Geometry: final body of the model. Coordinates: model frame, mm. A direction names the side the tool comes from. Coordinates: 2 decimals unless noted, no trailing zeros. Write each loop counter-clockwise with the first axis right and the second up, starting at its lowest first coordinate (ties: lowest second). Pieces come first, ordered by that corner, then holes. Notation, with made-up numbers: (-34, 11) - (-28, 11) arc R12 ccw to (-28, 22) - close; hole circle Ø10 at (38, -5.75). An arc over 180 degrees is marked (long way). Answer as a JSON object with one key per item and string values. Group by question number.
Item 1: Line query: line 1 along X through (y, z) = (175, 3.9); line 2 along Y through (x, z) = (166, 1.9); line 3 along Y through (x, z) = (156, 4.15). Output: solid intervals per line, ascending. Write a range as from..to.
Item 2: Mould query, pull axis X, two halves, no side actions, for faces 3 (the flat face through (-3, 167, 0)), 4 (the flat face through (16, -158, 3)). Classes: pulls with the +X half, pulls with the -X half, needs draft (parallel to the pull), parting line crosses it, or undercut.
Item 3: Section C-C on z = 3. State how many separate pieces and enclosed holes the cut face has, and give its area (3 significant figures).
Item 4: Section A-A on y = -11.5. Return loops of the section in (x, z), and give its area (3 significant figures).
Item 5: Set-up query: faces 1 (the flat face through (-16.892, -158.094, 2.958)), 2 (the flat face through (-3, 167, 6)). Return all of +Z, -Z, +X, -X, +Y, -Y with unobstructed straight access to the full face (end or side cutting, diameter ignored); none if empty.
Item 6: Section B-B on x = 90. Return loops of the section in (y, z).
Item 7: First-contact query: pin 1 Ø1.8 at (x, y) = (-176, -145) entering from -Z; pin 2 Ø3.5 at (x, y) = (-166, -165) entering from +Z; pin 3 Ø3 at (x, z) = (56, 3.5) entering from -Y. Flat tips, straight axial feed; report the tip coordinate or a pass-through.
```python
from build123d import *

# Parameters (mm, degrees)
F0_R     = 4
F0_R_2   = 1.5
F1_DEPTH = 6


with BuildPart() as f1:
    # F0 (on Top) → F1 (new body)
    with BuildSketch(Plane.XY):
        Polygon((185, 185), (-185, 185), (-185, -185), (-155, -185), (-145.34165, -182.651207), (145.154789, -182.651207), (155, -185), (185, -185), align=None)
        with Locations((-166, -175)):
            Circle(F0_R, mode=Mode.SUBTRACT)
        with Locations((-166, -165)):
            Circle(F0_R_2, mode=Mode.SUBTRACT)
        with Locations((-176, -145)):
            Circle(F0_R_2, mode=Mode.SUBTRACT)
        with Locations((-156, -145)):
            Circle(F0_R_2, mode=Mode.SUBTRACT)
        with Locations((166, -175)):
            Circle(F0_R, mode=Mode.SUBTRACT)
        with Locations((166, -164.2)):
            Circle(F0_R_2, mode=Mode.SUBTRACT)
        with Locations((156, -145)):
            Circle(F0_R_2, mode=Mode.SUBTRACT)
        with Locations((176, -145)):
            Circle(F0_R_2, mode=Mode.SUBTRACT)
        with BuildLine():
            ThreePointArc((-130, 142.348793), (-129.014539, 144.241247), (-127.020345, 145))
            Line((-127.020345, 145), (127.020345, 145))
            ThreePointArc((127.020345, 145), (129.014539, 144.241247), (130, 142.348793))
            Line((130, 142.348793), (130, -132))
            ThreePointArc((130, -132), (129.12132, -134.12132), (127, -135))
            Line((127, -135), (104, -135))
            ThreePointArc((104, -135), (102.658359, -135.316718), (101.6, -136.2))
            Line((101.6, -136.2), (95.6, -144.2))
            ThreePointArc((95.6, -144.2), (95.15395, -145.051317), (95, -146))
            Line((95, -146), (95, -165))
            ThreePointArc((95, -165), (90, -170), (85, -165))
            Line((85, -165), (85, -148))
            ThreePointArc((85, -148), (84.12132, -145.87868), (82, -145))
            Line((82, -145), (30.242641, -145))
            ThreePointArc((30.242641, -145), (29.09459, -145.228361), (28.12132, -145.87868))
            Line((28.12132, -145.87868), (4, -170))
            Line((4, -170), (-0.5, -170))
            Line((-0.5, -170), (-4.999919, -169.972975))
            Line((-4.999919, -169.972975), (-29.121436, -145.877533))
            ThreePointArc((-29.121436, -145.877533), (-30.094308, -145.228051), (-31.241609, -145))
            Line((-31.241609, -145), (-77, -145))
            ThreePointArc((-77, -145), (-79.12132, -145.87868), (-80, -148))
            Line((-80, -148), (-80, -164.2))
            ThreePointArc((-80, -164.2), (-85, -169.2), (-90, -164.2))
            Line((-90, -164.2), (-90, -145.2))
            ThreePointArc((-90, -145.2), (-90.15395, -144.251317), (-90.6, -143.4))
            Line((-90.6, -143.4), (-96, -136.2))
            ThreePointArc((-96, -136.2), (-97.058359, -135.316718), (-98.4, -135))
            Line((-98.4, -135), (-127, -135))
            ThreePointArc((-127, -135), (-129.12132, -134.12132), (-130, -132))
            Line((-130, -132), (-130, 142.348793))
        make_face(mode=Mode.SUBTRACT)
        with Locations((-176, 175)):
            Circle(F0_R_2, mode=Mode.SUBTRACT)
        with Locations((-156, 175)):
            Circle(F0_R_2, mode=Mode.SUBTRACT)
        with Locations((156, 175)):
            Circle(F0_R_2, mode=Mode.SUBTRACT)
        with Locations((176, 175)):
            Circle(F0_R_2, mode=Mode.SUBTRACT)
    extrude(amount=F1_DEPTH)


solid = f1.part
```
Checks:
{
 "1": {"line 1": "-185..-177.5, -174.5..-157.5, -154.5..154.5, 157.5..174.5, 177.5..185", "line 2": "-185..-179, -171..-165.7, -162.7..185", "line 3": "-185..-146.5, -143.5..173.5, 176.5..185"},
 "2": {"face 3": "needs draft", "face 4": "undercut"},
 "3": {"separate pieces": "1", "enclosed holes": "13", "area": "60,000 mm^2"},
 "4": {"outline": "(-185, 0) - (-130, 0) - (-130, 6) - (-185, 6) - close; (130, 0) - (185, 0) - (185, 6) - (130, 6) - close", "area": "660 mm^2"},
 "5": {"face 1": "+Z, -Z", "face 2": "+Z, +X, -X, +Y, -Y"},
 "6": {"outline": "(-182.65, 0) - (-170, 0) - (-170, 6) - (-182.65, 6) - close; (145, 0) - (185, 0) - (185, 6) - (145, 6) - close"},
 "7": {"pin 1": "through", "pin 2": "z = 6", "pin 3": "y = -182.65"}
}
